```python
from build123d import *

# Parameters (mm, degrees)
SKETCH1_R           = 2.032
BOSS_EXTRUDE1_DEPTH = 12.446
FILLET2_R           = 12.7
SKETCH2_R           = 2.032
BOSS_EXTRUDE2_DEPTH = 6.19125
FILLET7_R           = 10.16
FILLET8_R           = 1.27


with BuildPart() as part:
    # Sketch1 → Boss-Extrude1 (new, symmetric)
    with BuildSketch(Plane(origin=(0, 0, 0), x_dir=(1, 0, 0), z_dir=(0, 1, 0))):
        with BuildLine():
            Line((2.960934797, -4.512856233), (13.6525, 2.501997733))
            ThreePointArc((13.6525, 2.501997733), (5.644977773, 33.686754268), (27.6225, 57.215416983))
            ThreePointArc((27.6225, 57.215416983), (20.663418632, 58.118296563), (13.6525, 58.42))
            Line((13.6525, 58.42), (-5.3975, 58.42))
            Line((-5.3975, 58.42), (-5.3975, 0))
            ThreePointArc((-5.3975, 0), (-2.56430894, -4.749455328), (2.960934797, -4.512856233))
        make_face()
        with Locations(Location((0, 0, 0), (0, 0, 270))):
            Circle(SKETCH1_R, mode=Mode.SUBTRACT)
    extrude(amount=BOSS_EXTRUDE1_DEPTH, both=True)

    # Fillet2
    fillet2_edges = [part.edges().sort_by_distance(p)[0] for p in [
        (13.6525, 0, -2.501997733),
    ]]
    fillet(fillet2_edges, radius=FILLET2_R)

    # Sketch2 → Boss-Extrude2 (add, symmetric)
    with BuildSketch(Plane(origin=(0, 0, 0), x_dir=(1, 0, 0), z_dir=(0, 1, 0))):
        with BuildLine():
            Line((-5.3975, 40.64), (-14.492103254, 37.881269921))
            ThreePointArc((-14.492103254, 37.881269921), (-17.59286619, 35.227356842), (-17.740238368, 31.148598838))
            Line((-17.740238368, 31.148598838), (-5.3975, 0))
            Line((-5.3975, 0), (-5.3975, 40.64))
        make_face()
        with Locations(Location((-13.0175, 33.02, 0), (0, 0, 270))):
            Circle(SKETCH2_R, mode=Mode.SUBTRACT)
    extrude(amount=BOSS_EXTRUDE2_DEPTH, both=True)

    # Fillet7
    fillet7_edges = [part.edges().sort_by_distance(p)[0] for p in [
        (-5.3975, 0, -40.64),
    ]]
    fillet(fillet7_edges, radius=FILLET7_R)

    # Fillet8
    fillet8_edges = [part.edges().sort_by_distance(p)[0] for p in [
        (-5.3975, 0, -58.42),
        (27.6225, 0, -57.215416983),
    ]]
    fillet(fillet8_edges, radius=FILLET8_R)


solid = part.part
```
Work out the finished part from the listing and answer in its coordinate system (mm). A direction names the side the tool comes from. Give positions to 0.01 mm unless a question says otherwise; leave off trailing zeros. Loops run counter-clockwise (first coordinate to the right, second up) from the corner with the lowest first, then second, coordinate; pieces in that order, holes last. Notation, with made-up numbers: M -26,7 L -6,7 A24 cw -6,19 Z; hole C -11,-26 d1. An arc over 180 degrees is marked long. One line per item, written item: value. Start each with the question number.
1. Which of the six approach directions +Z, -Z, +X, -X, +Y, -Y give full straight-line access (tool end or side, diameter ignored) to faces 1 (the face through (-10, -6.191, -24)), 2 (the face through (-10, 6.191, -24)), 3 (the face through (-5.398, 8, -29))?
2. Find section B-B (z = -33.02). Give the vertices of the cut face in (x, y).
3. Find section D-D (y = -3). State how many separate pieces and enclosed holes the cut face has, and give its area (3 significant figures).
4. Find the intervals of material crossed by probe 1 along Y at (x, z) = (-9, -36.5); probe 2 along X at (y, z) = (7.75, -0.5); probe 3 along X at (y, z) = (-7.5, 0), in increasing order.
5. Determine the mould class of faces 4 (the face through (6.437, 0.174, -36.328)), 5 (the face through (-13.54, 0.09, -38.17)), 6 (the face through (8.264, 0.174, -2.536)), 7 (the face through (-11.655, 0.087, -15.792)) for opening direction Z: released by +Z, released by -Z, zero draft, split by the parting line, or undercut.
6. Find section C-C (z = -14). Give the vertices of the cut face in (x, y).
7. Each of these flat-tipped pins is pushed along its axis until it touches: P1, Ø12.5, axis at y = -2, z = -18.5, coming from the -X side; P2, Ø1.5, axis at y = -2, z = -20.5, coming from the +X side; P3, Ø10, axis at y = -8.5, z = -37.5, coming from the +X side; P4, Ø10, axis at x = -9.5, z = -26, coming from the -Y side. Where does it stop, or does it pass through?
8. Find section A-A (x = 0). Give the vertices of the cut face in (y, z).
Reported:
1. face 1: +Z, -Z, -X, -Y
1. face 2: +Z, -Z, -X, +Y
1. face 3: -Z, -X
2. outline: M -18.1,-6.19 L -15.05,-6.19 L -15.05,6.19 L -18.1,6.19 Z; M -10.99,-6.19 L -5.4,-6.19 L -5.4,-12.45 L 5.48,-12.45 L 5.48,12.45 L -5.4,12.45 L -5.4,6.19 L -10.99,6.19 Z
3. separate pieces: 1
3. enclosed holes: 2
3. area: 1,170 mm²
4. probe 1: y = -6.19 to 6.19
4. probe 2: x = -5.4 to -1.97, 1.97 to 7.46
4. probe 3: x = -5.4 to -2.03, 2.03 to 7.19
5. face 4: undercut
5. face 5: released by -Z
5. face 6: undercut
5. face 7: released by +Z
6. outline: M -10.95,-6.19 L -5.4,-6.19 L -5.4,-12.45 L 6.6,-12.45 L 6.6,12.45 L -5.4,12.45 L -5.4,6.19 L -10.95,6.19 Z
7. P1: stops at x = -15.2
7. P2: stops at x = 5.08
7. P3: stops at x = 9.3
7. P4: stops at y = -12.45
8. outline: M -12.45,-58.42 L 12.45,-58.42 L 12.45,-2.03 L -12.45,-2.03 Z; M -12.45,2.03 L 12.45,2.03 L 12.45,5.4 L -12.45,5.4 Z
